Source: CAD feature listing. Evaluate the final solid. Frame: model axes, mm. Round coordinates to 2 decimals unless told otherwise and drop trailing zeros. Write each loop counter-clockwise with the first axis right and the second up, starting at its lowest first coordinate (ties: lowest second). Pieces come first, ordered by that corner, then holes.
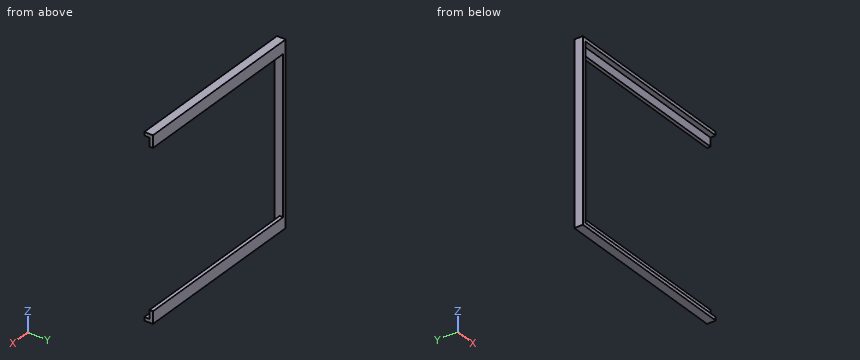
from build123d import *

# Parameters (mm, degrees)
F0_W      = 104
F0_H      = 104
F1_DEPTH  = 2
F2_W      = 104
F2_H      = 2
F3_DEPTH  = 3
F4_W      = 2
F4_H      = 102
F5_DEPTH  = 3
F6_W      = 102
F6_H      = 2
F7_DEPTH  = 3
F10_W     = 102
F10_H     = 90
F11_DEPTH = 25


with BuildPart() as f1:
    # F0 (on Front) → F1 (new body)
    with BuildSketch(Plane.XZ):
        Rectangle(F0_W, F0_H)
    extrude(amount=F1_DEPTH)

    # F2 (on face) → F3 (join)
    with BuildSketch(Plane.XZ.offset(2)):
        with Locations((0, 51)):
            Rectangle(F2_W, F2_H)
    extrude(amount=F3_DEPTH)

    # F4 (on face) → F5 (join)
    with BuildSketch(Plane.XZ.offset(2)):
        with Locations((-51, -1)):
            Rectangle(F4_W, F4_H)
    extrude(amount=F5_DEPTH)

    # F6 (on face) → F7 (join)
    with BuildSketch(Plane.XZ.offset(2)):
        with Locations((1, -51)):
            Rectangle(F6_W, F6_H)
    extrude(amount=F7_DEPTH)

    # F10 (on face) → F11 (cut)
    with BuildSketch(Plane.XZ.offset(2)):
        with Locations((1, 0)):
            Rectangle(F10_W, F10_H)
    extrude(amount=-F11_DEPTH, mode=Mode.SUBTRACT)


solid = f1.part
1) Contact query for flat-ended pins moving along their axis: P1, Ø1.5, axis at y = -2.5, z = 22.5, coming from the +X side; P2, Ø2.5, axis at x = 23.5, z = 47, coming from the -Y side. Output: stop coordinate, or through.
Taken from the geometry:
P1: stops at x = -50
P2: stops at y = -2
2) Section query B-B on y = -1. Return the cut outline in (x, z), then the cut area to 3 significant figures.
Taken from the geometry:
outline: (-52, -52) - (52, -52) - (52, -45) - (-50, -45) - (-50, 45) - (52, 45) - (52, 52) - (-52, 52) - close
area: 1,640 mm2
3) Section query C-C on z = 22.5. Return the cut outline in (x, y), then the cut area to 3 significant figures.
Taken from the geometry:
outline: (-52, -5) - (-50, -5) - (-50, 0) - (-52, 0) - close
area: 10.0 mm2
4) Material intervals for line 1 (Z direction, x = 23.5, y = -2.35); line 2 (Z direction, x = 21, y = -1.3); line 3 (X direction, y = -2.3, z = -14), sorted ascending.
Taken from the geometry:
line 1: z = -52 to -50, 50 to 52
line 2: z = -52 to -45, 45 to 52
line 3: x = -52 to -50
5) Section query A-A on x = -18. Return the cut outline in (y, z).
Taken from the geometry:
outline: (-5, -52) - (0, -52) - (0, -45) - (-2, -45) - (-2, -50) - (-5, -50) - close; (-5, 50) - (-2, 50) - (-2, 45) - (0, 45) - (0, 52) - (-5, 52) - close
